Check sheet for the modelled part. Datum: model origin and axes. Units: mm. A direction names the side the tool comes from. Round coordinates to 2 decimals unless told otherwise and drop trailing zeros. Write each loop counter-clockwise with the first axis right and the second up, starting at its lowest first coordinate (ties: lowest second). Pieces come first, ordered by that corner, then holes.
Item 1: Section check C-C, the plane x = 65. Record the cut outline in (y, z), plus the area to 3 significant figures.
Item 2: Release check for a two-part mould opening along Z. For faces 1 (the flat face through (44, 0, -7.5)), 2 (the flat face through (44, 0, -6)), 3 (the flat face through (44, 7.5, 0)) record: pulls with the +Z half, pulls with the -Z half, needs draft (parallel to the pull), parting line crosses it, or undercut.
Item 3: Material ranges on line 1 along Z through (x, y) = (67, 1); line 2 along Y through (x, z) = (33, -4.25); line 3 along Y through (x, z) = (85, 7), recorded low to high.
Item 4: Section check B-B, the plane y = 0. Record the cut outline in (x, z), plus the area to 3 significant figures.
Item 5: Set-up check for faces 4 (the flat face through (44, 0, 5.5)), 5 (the flat face through (44, 0, 7.5)): record each of +Z, -Z, +X, -X, +Y, -Y from which the full face is reachable in a straight line by a thin tool's end or side.
Item 6: Section check A-A, the plane z = -2.5. Record the cut outline in (x, y), plus the area to 3 significant figures.
Item 7: Depth check by flat-ended pin: pin 1 (2.5 mm diameter, centred on x = 65, y = 0, fed in from -Z). Enter the tip coordinate at first touch or a pass-through.
Item 8: Section check D-D, the plane y = 5. Record the cut outline in (x, z), plus the area to 3 significant figures.
from build123d import *

# Parameters (mm, degrees)
MEMBER_15_15_1_5_1_DEPTH = 90
SKETCH_3_R               = 1.5
CUT_EXTRUDE_1_DEPTH      = 92.549167118


with BuildPart() as part:
    # Sketch1 → Member 15 _15_ 1.5_1 (new body)
    with BuildSketch(Plane(origin=(0, 0, 0), x_dir=(0, 0, -1), z_dir=(1, 0, 0))):
        Polygon((-6, -7.5), (6, -7.5), (7.5, -7.5), (7.5, -6), (7.5, 6), (7.5, 7.5), (6, 7.5), (-6, 7.5), (-7.5, 7.5), (-7.5, 6), (-7.5, -6), (-7.5, -7.5), align=None)
        Polygon((-4, -6), (4, -6), (6, -6), (6, -3.5), (6, 3.5), (6, 6), (3.5, 6), (-3.5, 6), (-5.5, 6), (-5.5, 3.5), (-5.5, -3.5), (-5.5, -6), align=None, mode=Mode.SUBTRACT)
    extrude(amount=MEMBER_15_15_1_5_1_DEPTH)

    # 草图3 → 切除-拉伸1 (cut, through all)
    with BuildSketch(Plane.XY.offset(7.5)):
        with Locations((85, 0)):
            Circle(SKETCH_3_R)
        with Locations((65, 0)):
            Circle(SKETCH_3_R)
    extrude(amount=-CUT_EXTRUDE_1_DEPTH, mode=Mode.SUBTRACT)


solid = part.part
Values found:
1. outline: (-7.5, -7.5) - (-1.5, -7.5) - (-1.5, -6) - (-6, -6) - (-6, 5.5) - (-1.5, 5.5) - (-1.5, 7.5) - (-7.5, 7.5) - close; (1.5, -7.5) - (7.5, -7.5) - (7.5, 7.5) - (1.5, 7.5) - (1.5, 5.5) - (6, 5.5) - (6, -6) - (1.5, -6) - close
1. area: 76.5 mm2
2. face 1: pulls with the -Z half
2. face 2: undercut
2. face 3: needs draft
3. line 1: z = -7.5 to -6, 5.5 to 7.5
3. line 2: y = -7.5 to -6, 6 to 7.5
3. line 3: y = -7.5 to -1.5, 1.5 to 7.5
4. outline: (0, -7.5) - (63.5, -7.5) - (63.5, -6) - (0, -6) - close; (0, 5.5) - (63.5, 5.5) - (63.5, 7.5) - (0, 7.5) - close; (66.5, -7.5) - (83.5, -7.5) - (83.5, -6) - (66.5, -6) - close; (66.5, 5.5) - (83.5, 5.5) - (83.5, 7.5) - (66.5, 7.5) - close; (86.5, -7.5) - (90, -7.5) - (90, -6) - (86.5, -6) - close; (86.5, 5.5) - (90, 5.5) - (90, 7.5) - (86.5, 7.5) - close
4. area: 294 mm2
5. face 4: +X, -X
5. face 5: +Z, +X, -X, +Y, -Y
6. outline: (0, -7.5) - (90, -7.5) - (90, -6) - (0, -6) - close; (0, 6) - (90, 6) - (90, 7.5) - (0, 7.5) - close
6. area: 270 mm2
7. pin 1: passes through
8. outline: (0, -7.5) - (90, -7.5) - (90, -6) - (0, -6) - close; (0, 5.5) - (90, 5.5) - (90, 7.5) - (0, 7.5) - close
8. area: 315 mm2
